Design review of the part built by this model. Coordinates are the model's own, in mm. Face numbers are marked on the shaded views. A direction names the side the tool comes from. Round coordinates to 2 decimals unless told otherwise and drop trailing zeros. Write each loop counter-clockwise with the first axis right and the second up, starting at its lowest first coordinate (ties: lowest second). Pieces come first, ordered by that corner, then holes. Notation, with made-up numbers: M 60,-2.75 L 100,-2.75 A15 ccw 100,10.25 Z; hole C 88.5,-23.5 d4. An arc over 180 degrees is marked long. One line per question, with ' | ' between items. Start each with the question number.
Item 1: For L1, parallel to Z at x = 40, y = 6; L2, parallel to X at y = 7.3, z = -15; L3, parallel to X at y = 8.5, z = -16.5, list the stretches that pass through material, from the lowest coordinate up.
Item 2: Add section C-C, the plane y = 40. State the section outline as (x, z) points.
Item 3: Add section B-B, the plane x = 40. State the section outline as (y, z) points (3 decimals).
Item 4: Add section A-A, the plane z = 0. State the section outline as (x, y) points.
Item 5: Add section D-D, the plane x = -180.5. State the section outline as (y, z) points.
Item 6: Insertion check: pin 1 Ø1 at (y, z) = (30.5, 4.5) entering from -X; pin 2 Ø8 at (y, z) = (39, 7) entering from -X; pin 3 Ø7 at (x, z) = (20, -15) entering from +Y; pin 4 Ø12 at (y, z) = (18, 18.5) entering from +X. Each pin has a flat end and moves straight along its axis. Give the tip position at first contact, or say it passes through.
Item 7: Machinability: for the marked faces 1, 2 and 3, which of the approach directions +Z, -Z, +X, -X, +Y, -Y give a long, thin tool a straight path to every point of the face, cutting with its end or side? Answer none if there is none.
```python
from build123d import *

# Parameters (mm, degrees)
SKETCH1_W           = 100
SKETCH1_H           = 50
BOSS_EXTRUDE1_DEPTH = 10
SKETCH8_W           = 150
SKETCH8_H           = 50
BOSS_EXTRUDE3_DEPTH = 10
SKETCH10_R          = 12.5
BOSS_EXTRUDE4_DEPTH = 5
SKETCH12_R          = 10.05
BOSS_EXTRUDE5_DEPTH = 30
SKETCH13_W          = 40
SKETCH13_H          = 50
CUT_EXTRUDE3_DEPTH  = 5
FILLET1_R           = 10


# Read off the part's stored shape, not the designer's step: M5 Clearance Hole1
with BuildPart() as part:
    # Sketch1 → Boss-Extrude1 (new body)
    with BuildSketch(Plane(origin=(0, 0, 0), x_dir=(1, 0, 0), z_dir=(0, 1, 0))):
        Rectangle(SKETCH1_W, SKETCH1_H)
    extrude(amount=BOSS_EXTRUDE1_DEPTH)

    # Sketch8 → Boss-Extrude3 (add)
    with BuildSketch(Plane(origin=(0, 10, 0), x_dir=(1, 0, 0), z_dir=(0, 1, 0))):
        with Locations((-125, 0)):
            Rectangle(SKETCH8_W, SKETCH8_H)
    extrude(amount=-BOSS_EXTRUDE3_DEPTH)

    # Sketch10 → Boss-Extrude4 (add)
    with BuildSketch(Plane(origin=(0, 10, 0), x_dir=(1, 0, 0), z_dir=(0, 1, 0))):
        with Locations(Location((-25, 0, 0), (0, 0, 270))):
            Circle(SKETCH10_R)
    extrude(amount=BOSS_EXTRUDE4_DEPTH)

    # Sketch12 → Boss-Extrude5 (add)
    with BuildSketch(Plane(origin=(0, 15, 0), x_dir=(1, 0, 0), z_dir=(0, 1, 0))):
        with Locations(Location((-25, 0, 0), (0, 0, 270))):
            Circle(SKETCH12_R)
    extrude(amount=BOSS_EXTRUDE5_DEPTH)

    # Sketch13 → Cut-Extrude3 (cut)
    with BuildSketch(Plane.XZ):
        with Locations((30, 0)):
            Rectangle(SKETCH13_W, SKETCH13_H)
    extrude(amount=-CUT_EXTRUDE3_DEPTH, mode=Mode.SUBTRACT)

    # M5 Clearance Hole1 outline → M5 Clearance Hole1 (revolve, cut)
    with BuildSketch(Plane(origin=(20, 0, -15), x_dir=(1, 0, 0), z_dir=(0, 0, 1))):
        Polygon((2.75, 5.025), (2.75, 10), (0, 10), (0, 5), (2.775, 5), align=None)
    revolve(axis=Axis((20, 0, -15), (0, 1, 0)), mode=Mode.SUBTRACT)

    # M5 Clearance Hole1 2 outline → M5 Clearance Hole1 2 (revolve, cut)
    with BuildSketch(Plane(origin=(20, 0, 15), x_dir=(1, 0, 0), z_dir=(0, 0, 1))):
        Polygon((2.75, 5.025), (2.75, 10), (0, 10), (0, 5), (2.775, 5), align=None)
    revolve(axis=Axis((20, 0, 15), (0, 1, 0)), mode=Mode.SUBTRACT)

    # M5 Clearance Hole1 3 outline → M5 Clearance Hole1 3 (revolve, cut)
    with BuildSketch(Plane(origin=(40, 0, 15), x_dir=(1, 0, 0), z_dir=(0, 0, 1))):
        Polygon((2.75, 5.025), (2.75, 10), (0, 10), (0, 5), (2.775, 5), align=None)
    revolve(axis=Axis((40, 0, 15), (0, 1, 0)), mode=Mode.SUBTRACT)

    # M5 Clearance Hole1 4 outline → M5 Clearance Hole1 4 (revolve, cut)
    with BuildSketch(Plane(origin=(40, 0, -15), x_dir=(1, 0, 0), z_dir=(0, 0, 1))):
        Polygon((2.75, 5.025), (2.75, 10), (0, 10), (0, 5), (2.775, 5), align=None)
    revolve(axis=Axis((40, 0, -15), (0, 1, 0)), mode=Mode.SUBTRACT)

    # Fillet1
    fillet1_edges = [part.edges().sort_by_distance(p)[0] for p in [
        (-200, 5, -25),
        (-200, 5, 25),
    ]]
    fillet(fillet1_edges, radius=FILLET1_R)


solid = part.part
```
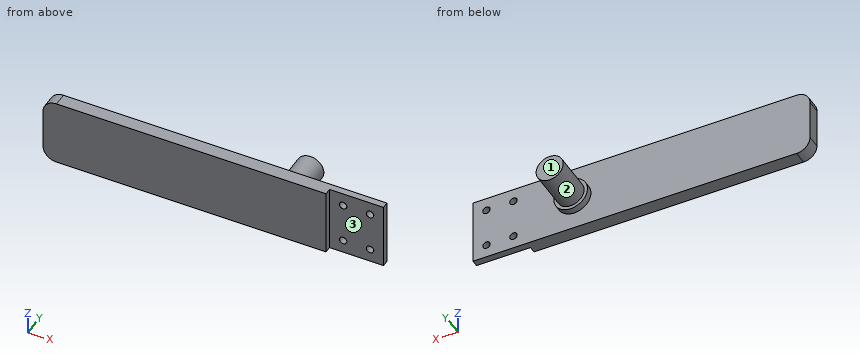
Computed values:
1) L1: z = -25 to -17.75, -12.25 to 12.25, 17.75 to 25 | L2: x = -200 to 17.25, 22.75 to 37.25, 42.75 to 50 | L3: x = -199.89 to 17.7, 22.3 to 37.7, 42.3 to 50
2) outline: C -25,0 d20.1
3) outline: M 5,-25 L 10,-25 L 10,-17.75 L 5.025,-17.75 L 5,-17.775 Z; M 5,-12.225 L 5.025,-12.25 L 10,-12.25 L 10,12.25 L 5.025,12.25 L 5,12.225 Z; M 5,17.775 L 5.025,17.75 L 10,17.75 L 10,25 L 5,25 Z
4) outline: M -200,0 L 10,0 L 10,5 L 50,5 L 50,10 L -12.5,10 L -12.5,15 L -14.95,15 L -14.95,45 L -35.05,45 L -35.05,15 L -37.5,15 L -37.5,10 L -200,10 Z
5) outline: M 0,-25 L 10,-25 L 10,25 L 0,25 Z
6) pin 1: stops at x = -34.22 | pin 2: stops at x = -34.59 | pin 3: stops at y = 10 | pin 4: passes through
7) face 1: +Z, -Z, +X, -X, +Y | face 2: +Y | face 3: +Z, -Z, +X, -Y
